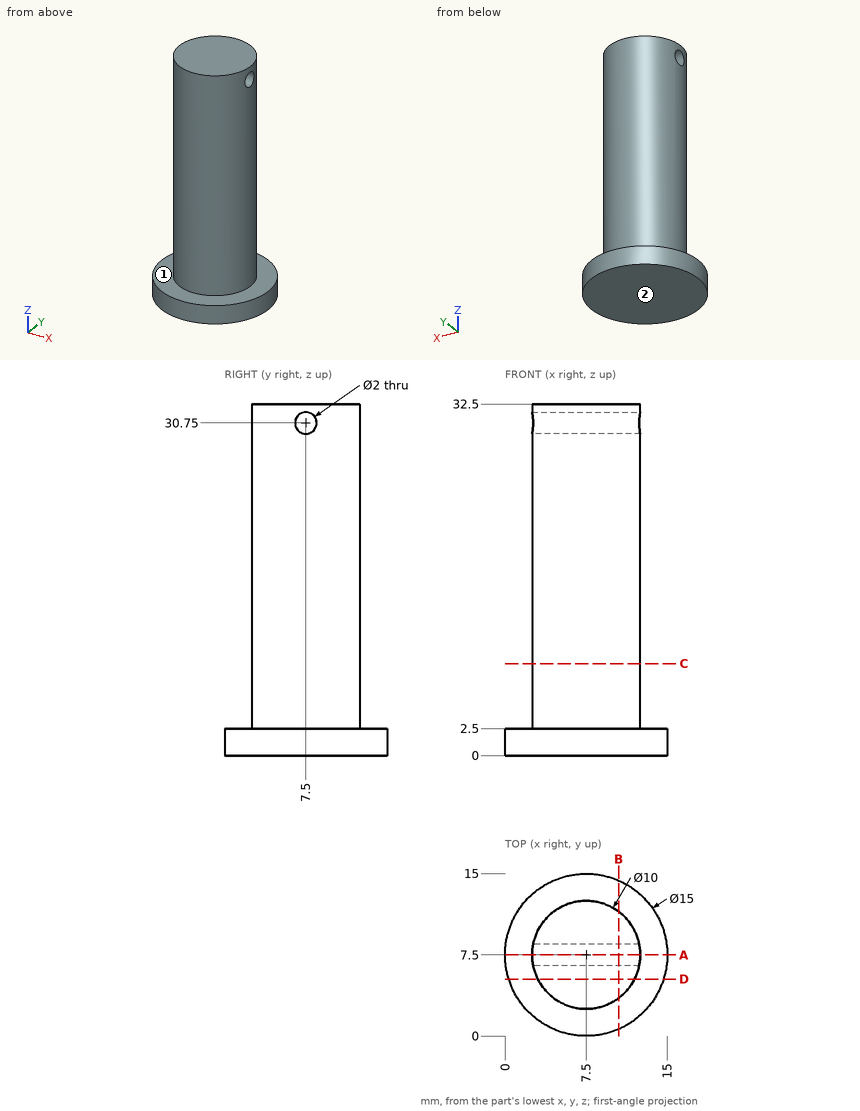
Source: three-view drawing plus pictorial views. Frame: mm from the lowest corner of the part. A direction names the side the tool comes from. Round coordinates to 2 decimals unless told otherwise and drop trailing zeros. Loops run counter-clockwise (first coordinate to the right, second up) from the corner with the lowest first, then second, coordinate; pieces in that order, holes last.
1. Section query D-D on y = 5.25. Output: boundary loops of the cut face in (x, z), and give its area (3 significant figures).
2. Contact query for flat-ended pins moving along their axis: pin 1 (4 mm diameter, centred on x = 8.5, z = 27.5, fed in from -Y); pin 2 (1.6 mm diameter, centred on y = 7.5, z = 30.75, fed in from +X); pin 3 (3 mm diameter, centred on x = 10.5, y = 11, fed in from -Z); pin 4 (5 mm diameter, centred on x = 4.5, z = 7.5, fed in from +Y). Output: stop coordinate, or through.
3. Section query B-B on x = 10.5. Output: boundary loops of the cut face in (y, z).
4. Ray query, L1, parallel to Z at x = 7.5, y = 7.5; L2, parallel to Z at x = 13, y = 9.75; L3, parallel to Y at x = 8.25, z = 30.75. Return the intervals inside material, ascending.
5. Section query A-A on y = 7.5. Output: boundary loops of the cut face in (x, z), and give its area (4 significant figures).
6. Section query C-C on z = 8.5. Output: boundary loops of the cut face in (x, y), and give its area (3 significant figures).
7. Access query for the marked faces 1 and 2. Directions: +Z, -Z, +X, -X, +Y, -Y. A direction counts if a zero-diameter tool reaches every point of the face in a straight line with its end or side. Return the directions, or none.
Answers below:
1. outline: (0.35, 0) - (14.65, 0) - (14.65, 2.5) - (11.97, 2.5) - (11.97, 32.5) - (3.03, 32.5) - (3.03, 2.5) - (0.35, 2.5) - close
1. area: 304 mm2
2. pin 1: stops at y = 2.5
2. pin 2: passes through
2. pin 3: stops at z = 0
2. pin 4: stops at y = 12.47
3. outline: (0.63, 0) - (14.37, 0) - (14.37, 2.5) - (11.5, 2.5) - (11.5, 32.5) - (3.5, 32.5) - (3.5, 2.5) - (0.63, 2.5) - close; hole circle Ø2 at (7.5, 30.75)
4. L1: z = 0 to 29.75, 31.75 to 32.5
4. L2: z = 0 to 2.5
4. L3: y = 2.56 to 6.5, 8.5 to 12.44
5. outline: (0, 0) - (15, 0) - (15, 2.5) - (12.5, 2.5) - (12.5, 29.75) - (2.5, 29.75) - (2.5, 2.5) - (0, 2.5) - close; (2.5, 31.75) - (12.5, 31.75) - (12.5, 32.5) - (2.5, 32.5) - close
5. area: 317.5 mm2
6. outline: circle Ø10 at (7.5, 7.5)
6. area: 78.5 mm2
7. face 1: +Z
7. face 2: -Z, +X, -X, +Y, -Y
